The model under review builds one solid part; all positions refer to its coordinate system, in mm. A direction names the side the tool comes from. Give positions to 0.01 mm unless a question says otherwise; leave off trailing zeros. Loops run counter-clockwise (first coordinate to the right, second up) from the corner with the lowest first, then second, coordinate; pieces in that order, holes last. Notation, with made-up numbers: M 5,85 L 12,85 A16 cw 12,98 Z; hole C -14,79.25 d4. An arc over 180 degrees is marked long. One line per item, written item: value. Start each with the question number.
Q1. We need section C-C on x = -234. Write out the cut boundary in (y, z).
Q2. We need section D-D on z = 232. Write out the cut boundary in (x, y), plus the area to 3 significant figures.
Q3. For faces 1 (the face through (-191, -23.32, -62)), 2 (the face through (161.35, -34.66, 163.92)), list the 3-axis set-ups (+Z, -Z, +X, -X, +Y, -Y) from which the entire face can be reached by the end or side of a thin tool; tool diameter is ignored.
Q4. We need section A-A on y = -38. Give the number of separate pieces and of enclosed holes in the cut face, plus the area to 3 significant figures.
Q5. We need section B-B on y = -5. Write out the cut boundary in (x, z), plus the area to 3 significant figures.
Q6. To check wall thickness, follow line 1 along X through (y, z) = (15.5, 0); line 2 along Z through (x, y) = (11, -33); line 3 along X through (y, z) = (13, 19.5). State the ranges of each line that lie inside material, in increasing order. Write a range as from..to.
Q7. For pin 1 (5 mm diameter, centred on y = -34, z = -185, fed in from -X); pin 2 (5 mm diameter, centred on x = 149.5, y = -34.5, fed in from -Z); pin 3 (1 mm diameter, centred on x = 55.5, y = -0.5, fed in from -Z); pin 4 (4 mm diameter, centred on x = 12, z = 19, fed in from +Y), all flat-tipped, find the tip position at first contact; note any pin that passes through.
Autodesk Inventor part; units mm, degrees
ref_plane "YZ Plane" through (0, 0, 0) normal (1, 0, 0) x (0, 1, 0)
ref_plane "XZ Plane" through (0, 0, 0) normal (0, 1, 0) x (-1, 0, 0)
ref_plane "XY Plane" through (0, 0, 0) normal (0, 0, 1) x (1, 0, 0)
sketch "Esquisse2" plane through (0, 0, 0) normal (1, 0, 0) x (0, 1, 0)
  line L0 (-23.32, 215.2) -> (-23.32, 200.2)
  line L1 (-23.32, 200.2) -> (20.32, 200.2)
  spline S0 degree 4 poles (20.32, 200.2) (20.32, 180.2) (23.32, 170.4614) (34.7283, 130.1649) (37.5, 42) (37.5, 32) knots 1 1 1 1 1 2 3 3 3 3 3
  line L2 (37.5, 32) -> (37.5, 0)
  line L3 (-23.32, 200.2) -> (-23.32, 0)
  line L4 (-23.32, 0) -> (37.5, 0)
  line L5 (-36.3967, 0) -> (55.14, 0)
  point P0 (0, 0)
revolve "Révolution1" add sketch "Esquisse2" angle 360 about axis through (0, -10, 0) along (0, 1, 0)
sketch "Esquisse3" plane through (0, -23.32, 0) normal (0, -1, 0) x (1, 0, 0)
  circle A0 centre (-254.2, 0) radius 4
  circle A1 centre (254.2, 0) radius 4
  circle A2 centre (-20, -253.412) radius 4
  circle A3 centre (20, -253.412) radius 4
  circle A4 centre (-20, 253.412) radius 4
  circle A5 centre (20, 253.412) radius 4
  circle A6 centre (-22, 0) radius 2.5
  circle A7 centre (-11, 19.0526) radius 2.5
  circle A8 centre (11, 19.0526) radius 2.5
  circle A9 centre (22, 0) radius 2.5
  circle A10 centre (11, -19.0526) radius 2.5
  circle A11 centre (-11, -19.0526) radius 2.5
  line L0 (70.7107, 254.5584) -> (254.5584, 70.7107)
  arc A12 (254.5584, -70.7107) -> (254.5584, 70.7107) centre (183.8478, 0) ccw
  line L1 (254.5584, -70.7107) -> (70.7107, -254.5584)
  arc A13 (-70.7107, -254.5584) -> (70.7107, -254.5584) centre (0, -183.8478) ccw
  line L2 (-70.7107, -254.5584) -> (-254.5584, -70.7107)
  arc A14 (-254.5584, 70.7107) -> (-254.5584, -70.7107) centre (-183.8478, 0) ccw
  line L3 (-254.5584, 70.7107) -> (-70.7107, 254.5584)
  arc A15 (70.7107, 254.5584) -> (-70.7107, 254.5584) centre (0, 183.8478) ccw
extrude "Extrusion1" add sketch "Esquisse3" along normal blind 23
sketch "Esquisse6" plane through (0, 37.5, 0) normal (0, 1, 0) x (1, 0, 0)
  circle A0 centre (20, -253.412) radius 4
  circle A1 centre (-20, -253.412) radius 4
  circle A2 centre (20, 253.412) radius 4
  circle A3 centre (-20, 253.412) radius 4
  circle A4 centre (254.2, 0) radius 4
  circle A5 centre (-254.2, 0) radius 4
  circle A6 centre (-11, 19.0526) radius 2.5
  circle A7 centre (11, 19.0526) radius 2.5
  circle A8 centre (22, 0) radius 2.5
  circle A9 centre (11, -19.0526) radius 2.5
  circle A10 centre (-11, -19.0526) radius 2.5
  circle A11 centre (-22, 0) radius 2.5
  line L0 (254.5584, -70.7107) -> (70.7107, -254.5584)
  arc A12 (-70.7107, -254.5584) -> (70.7107, -254.5584) centre (0, -183.8478) ccw
  line L1 (-70.7107, -254.5584) -> (-254.5584, -70.7107)
  arc A13 (-254.5584, 70.7107) -> (-254.5584, -70.7107) centre (-183.8478, 0) ccw
  line L2 (-254.5584, 70.7107) -> (-70.7107, 254.5584)
  arc A14 (70.7107, 254.5584) -> (-70.7107, 254.5584) centre (0, 183.8478) ccw
  line L3 (70.7107, 254.5584) -> (254.5584, 70.7107)
  arc A15 (254.5584, -70.7107) -> (254.5584, 70.7107) centre (183.8478, 0) ccw
  point P0 (0, -32)
extrude "Extrusion3" cut sketch "Esquisse6" against normal blind 35 contours A6 | A7 | A8 | A9 | A10 | A11
properties part number "wheel_rim_mold_C"
Solved:
1. outline: M -46.32,-91.27 L -23.32,-91.27 L -23.32,91.27 L -46.32,91.27 Z
2. outline: M -93.27,-46.32 L 93.27,-46.32 L 93.27,-23.32 L -93.27,-23.32 Z
2. area: 4,290 mm2
3. face 1: +Y
3. face 2: +Z, +X, +Y, -Y
4. separate pieces: 1
4. enclosed holes: 12
4. area: 203,000 mm2
5. outline: C 0,0 d400.4
5. area: 126,000 mm2
6. line 1: -200.2..-24.5, -19.5..19.5, 24.5..200.2
6. line 2: -283.24..-21.55, -16.55..16.55, 21.55..283.24
6. line 3: -199.25..-13.46, -8.54..8.54, 13.46..199.25
7. pin 1: x = -142.77
7. pin 2: z = -178.27
7. pin 3: z = -192.5
7. pin 4: y = 37.5
